Design review of the part built by this model. Coordinates are the model's own, in mm. Give positions to 0.01 mm unless a question says otherwise; leave off trailing zeros. Order: outer loops, then holes, each group sorted by start corner. A loop starts at its lowest first (then second) coordinate and runs counter-clockwise, first axis right, second up. Notation, with made-up numbers: (52, 22.25) -> (99, 22.25) arc R20 ccw to (99, 42.25) -> close; hole circle Ø10 at (5, -35.5). An arc over 180 degrees is marked (long way). Return JSON: item names as keys, results as strings.
```python
from build123d import *

# Parameters (mm, degrees)
SKETCH_3_R          = 1
EXTRUDE_3_DEPTH     = 2
SKETCH_4_R          = 1
CUT_EXTRUDE_2_DEPTH = 2
SKETCH_6_R          = 1.25
CUT_EXTRUDE_6_DEPTH = 2
SKETCH_7_R          = 1
CUT_EXTRUDE_7_DEPTH = 10
SKETCH_8_W          = 4
SKETCH_8_H          = 2
EXTRUDE_6_DEPTH     = 2
CUT_EXTRUDE_8_DEPTH = 2


with BuildPart() as part:
    # 草圖3 → 填料-伸長3 (new body)
    with BuildSketch(Plane.XY):
        Polygon((1, 40), (0, 40), (0, 39), (0, 1), (0, 0), (1, 0), (113, 0), (114, 0), (114, 1), (114, 39), (114, 40), (113, 40), align=None)
        with Locations((4, 24)):
            Circle(SKETCH_3_R, mode=Mode.SUBTRACT)
        with Locations((4, 16)):
            Circle(SKETCH_3_R, mode=Mode.SUBTRACT)
        with Locations(Location((110, 16, 0), (0, 0, 180))):
            Circle(SKETCH_3_R, mode=Mode.SUBTRACT)
        with Locations(Location((110, 24, 0), (0, 0, 180))):
            Circle(SKETCH_3_R, mode=Mode.SUBTRACT)
    extrude(amount=EXTRUDE_3_DEPTH)

    # 草圖4 → 除料-伸長2 (cut)
    with BuildSketch(Plane.XY.offset(2)):
        with Locations((40, 24)):
            Circle(SKETCH_4_R)
        with Locations((40, 16)):
            Circle(SKETCH_4_R)
        with Locations(Location((74, 16, 0), (0, 0, 180))):
            Circle(SKETCH_4_R)
        with Locations(Location((74, 24, 0), (0, 0, 180))):
            Circle(SKETCH_4_R)
    extrude(amount=-CUT_EXTRUDE_2_DEPTH, mode=Mode.SUBTRACT)

    # 草圖6 → 除料-伸長6 (cut)
    with BuildSketch(Plane.XY.offset(2)):
        with Locations((41, 33)):
            Circle(SKETCH_6_R)
        with Locations((73, 33)):
            Circle(SKETCH_6_R)
        with Locations((73, 7)):
            Circle(SKETCH_6_R)
        with Locations((41, 7)):
            Circle(SKETCH_6_R)
    extrude(amount=-CUT_EXTRUDE_6_DEPTH, mode=Mode.SUBTRACT)

    # 草圖7 → 除料-伸長7 (cut)
    with BuildSketch(Plane.XY.offset(2)):
        with Locations((22, 38)):
            Circle(SKETCH_7_R)
        with Locations((92, 38)):
            Circle(SKETCH_7_R)
        with Locations((92, 2)):
            Circle(SKETCH_7_R)
        with Locations((22, 2)):
            Circle(SKETCH_7_R)
    extrude(amount=-CUT_EXTRUDE_7_DEPTH, mode=Mode.SUBTRACT)

    # 草圖8 → 填料-伸長6 (add)
    with BuildSketch(Plane.XY.offset(2)):
        with Locations((22, 41)):
            Rectangle(SKETCH_8_W, SKETCH_8_H)
        with Locations((22, -1)):
            Rectangle(SKETCH_8_W, SKETCH_8_H)
        with Locations((92, -1)):
            Rectangle(SKETCH_8_W, SKETCH_8_H)
        with Locations((92, 41)):
            Rectangle(SKETCH_8_W, SKETCH_8_H)
    extrude(amount=-EXTRUDE_6_DEPTH)

    # 草圖9 → 除料-伸長8 (cut)
    with BuildSketch(Plane.XY.offset(2)):
        with BuildLine():
            Line((0, 22), (2, 22))
            ThreePointArc((2, 22), (2.707106781, 21.707106781), (3, 21))
            Line((3, 21), (3, 19))
            ThreePointArc((3, 19), (2.707106781, 18.292893219), (2, 18))
            Line((2, 18), (0, 18))
            Line((0, 18), (0, 22))
        make_face()
        with BuildLine():
            Line((18, 40), (20, 40))
            ThreePointArc((20, 40), (19, 39), (18, 40))
        make_face()
        with BuildLine():
            Line((24, 40), (26, 40))
            ThreePointArc((26, 40), (25, 39), (24, 40))
        make_face()
        with BuildLine():
            Line((18, 0), (20, 0))
            ThreePointArc((20, 0), (19, 1), (18, 0))
        make_face()
        with BuildLine():
            Line((24, 0), (26, 0))
            ThreePointArc((26, 0), (25, 1), (24, 0))
        make_face()
        with BuildLine():
            Line((90, 0), (88, 0))
            ThreePointArc((88, 0), (89, 1), (90, 0))
        make_face()
        with BuildLine():
            Line((96, 0), (94, 0))
            ThreePointArc((94, 0), (95, 1), (96, 0))
        make_face()
        with BuildLine():
            Line((90, 40), (88, 40))
            ThreePointArc((88, 40), (89, 39), (90, 40))
        make_face()
        with BuildLine():
            Line((111, 21), (111, 19))
            ThreePointArc((111, 19), (111.292893219, 18.292893219), (112, 18))
            Line((112, 18), (114, 18))
            Line((114, 18), (114, 22))
            Line((114, 22), (112, 22))
            ThreePointArc((112, 22), (111.292893219, 21.707106781), (111, 21))
        make_face()
        with BuildLine():
            Line((96, 40), (94, 40))
            ThreePointArc((94, 40), (95, 39), (96, 40))
        make_face()
    extrude(amount=-CUT_EXTRUDE_8_DEPTH, mode=Mode.SUBTRACT)


solid = part.part
```
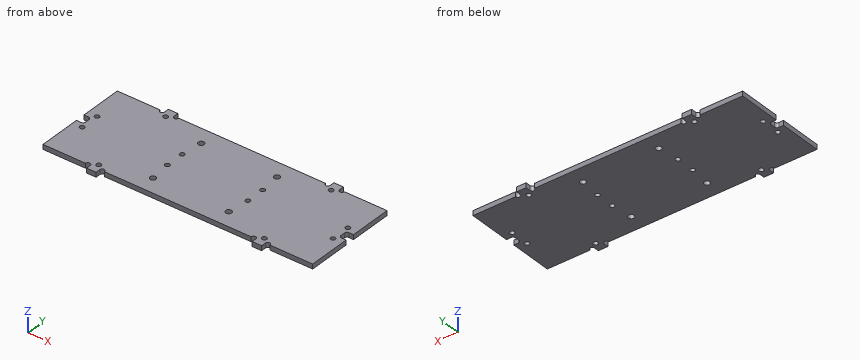
Item 1: Add section C-C (z = 1.45). Give the number of separate pieces and of enclosed holes in the cut face, plus the area to 3 significant figures.
Result set:
{"separate pieces": "1", "enclosed holes": "16", "area": "4,500 mm^2"}
Item 2: Wall thickness on L1, parallel to Y at x = 4, z = 0.9; L2, parallel to Y at x = 92, z = 0.1; L3, parallel to Y at x = 74, z = 1.6: over which ranges is each line inside the solid? List them lowest first. Write a range as [from, to].
Result set:
{"L1": "y = [0, 15], [17, 23], [25, 40]", "L2": "y = [-2, 1], [3, 37], [39, 42]", "L3": "y = [0, 6.25], [7.75, 15], [17, 23], [25, 32.25], [33.75, 40]"}
Item 3: For pin 1 (0.6 mm diameter, centred on y = -1.5, z = 1, fed in from +X); pin 2 (1 mm diameter, centred on x = 113, z = 1.5, fed in from +Y); pin 3 (0.6 mm diameter, centred on x = 63.5, z = 1.5, fed in from -Y), all flat-tipped, find the tip position at first contact; note any pin that passes through.
Result set:
{"pin 1": "stops at x = 94", "pin 2": "stops at y = 40", "pin 3": "stops at y = 0"}
Item 4: Add section A-A (x = 110). Give the boundary of the cut face in (y, z), plus the area to 3 significant figures.
Result set:
{"outline": "(0, 0) -> (15, 0) -> (15, 2) -> (0, 2) -> close; (17, 0) -> (23, 0) -> (23, 2) -> (17, 2) -> close; (25, 0) -> (40, 0) -> (40, 2) -> (25, 2) -> close", "area": "72.0 mm^2"}
Item 5: Add section D-D (x = 95). Give the boundary of the cut face in (y, z).
Result set:
{"outline": "(1, 0) -> (39, 0) -> (39, 2) -> (1, 2) -> close"}
Item 6: Add section B-B (y = 2). Give the boundary of the cut face in (x, z).
Result set:
{"outline": "(0, 0) -> (21, 0) -> (21, 2) -> (0, 2) -> close; (23, 0) -> (91, 0) -> (91, 2) -> (23, 2) -> close; (93, 0) -> (114, 0) -> (114, 2) -> (93, 2) -> close"}
